```python
from build123d import *

# Parameters (mm, degrees)
SKETCH1_R            = 15
BOSS_EXTRUDE1_DEPTH  = 40
SKETCH2_R            = 35
BOSS_EXTRUDE2_DEPTH  = 5
SKETCH3_R            = 5
CUT_EXTRUDE1_DEPTH   = 64.639610307
CUT_EXTRUDE2_DEPTH   = 10
SKETCH5_W            = 7.5
SKETCH5_H            = 12
CUT_EXTRUDE3_DEPTH   = 64.639610307
M5_CLEARANCE_HOLE1_D = 5.5
CUT_EXTRUDE4_DEPTH   = 64.639610307


with BuildPart() as part:
    # Sketch1 → Boss-Extrude1 (new body)
    with BuildSketch(Plane.XY):
        Circle(SKETCH1_R)
    extrude(amount=BOSS_EXTRUDE1_DEPTH)

    # Sketch2 → Boss-Extrude2 (add)
    with BuildSketch(Plane(origin=(0, 0, 0), x_dir=(-1, 0, 0), z_dir=(0, 0, -1))):
        Circle(SKETCH2_R)
    extrude(amount=-BOSS_EXTRUDE2_DEPTH)

    # Sketch3 → Cut-Extrude1 (cut, through all)
    with BuildSketch(Plane(origin=(0, 0, 0), x_dir=(-1, 0, 0), z_dir=(0, 0, -1))):
        Circle(SKETCH3_R)
    extrude(amount=-CUT_EXTRUDE1_DEPTH, mode=Mode.SUBTRACT)

    # Sketch4 → Cut-Extrude2 (cut)
    with BuildSketch(Plane(origin=(0, 0, 0), x_dir=(-1, 0, 0), z_dir=(0, 0, -1))):
        Polygon((8, 0), (4, 6.92820323), (-4, 6.92820323), (-8, 0), (-4, -6.92820323), (4, -6.92820323), align=None)
    extrude(amount=-CUT_EXTRUDE2_DEPTH, mode=Mode.SUBTRACT)

    # Sketch5 → Cut-Extrude3 (cut, symmetric)
    with BuildSketch(Plane(origin=(0, 0, 0), x_dir=(1, 0, 0), z_dir=(0, 1, 0))):
        with Locations((11.25, -34)):
            Rectangle(SKETCH5_W, SKETCH5_H)
    cut_extrude3 = extrude(amount=CUT_EXTRUDE3_DEPTH, both=True, mode=Mode.SUBTRACT)

    # Mirror1: Cut-Extrude3 across plane
    add(cut_extrude3.mirror(Plane(origin=(0, 0, 0), x_dir=(0, 0, 1), z_dir=(1, 0, 0))), mode=Mode.SUBTRACT)

    # M5 Clearance Hole1 (through all)
    with Locations(Plane(origin=(0, 0, 0), x_dir=(-1, 0, 0), z_dir=(0, 0, -1))):
        with Locations((0, 27.5), (-27.5, 0), (27.5, 0), (0, -27.5)):
            Hole(M5_CLEARANCE_HOLE1_D / 2)

    # Sketch8 → Cut-Extrude4 (cut, through all)
    with BuildSketch(Plane(origin=(0, 0, 0), x_dir=(-1, 0, 0), z_dir=(0, 0, -1))):
        with BuildLine():
            Line((-34.957538249, -1.723519533), (1.723519533, 34.957538249))
            ThreePointArc((1.723519533, 34.957538249), (-24.748737342, 24.748737342), (-34.957538249, -1.723519533))
        make_face()
    extrude(amount=-CUT_EXTRUDE4_DEPTH, mode=Mode.SUBTRACT)


solid = part.part
```
Read the model definition and answer for the solid it produces. Units are mm, in the model's axes. A direction names the side the tool comes from. Coordinates: 2 decimals unless noted, no trailing zeros. Loops run counter-clockwise (first coordinate to the right, second up) from the corner with the lowest first, then second, coordinate; pieces in that order, holes last. Notation, with made-up numbers: (-28.75, 15.25) - (-24.75, 15.25) arc R16 cw to (-24.75, 24.25) - close; hole circle Ø11 at (80.5, 3). An arc over 180 degrees is marked (long way). Answer in a Markdown table with one row per item.
1. Given pin 1 (4 mm diameter, centred on y = 17, z = 4, fed in from +X); pin 2 (3 mm diameter, centred on y = 2, z = 24.5, fed in from +X); pin 3 (6 mm diameter, centred on x = 13, y = 5, fed in from +Z), each flat-ended and moving along its own axis, determine where each tip first touches the part or whether it passes through.
Conclusion:
| item | result |
|---|---|
| pin 1 | stops at x = 18.23 |
| pin 2 | stops at x = 14.99 |
| pin 3 | stops at z = 28 |
2. Straight lines are drawn through the part: line 1 (Y direction, x = 0, z = 4); line 2 (Z direction, x = -18, y = 18); line 3 (X direction, y = -4, z = 14). For each, find the intervals that lie inside material, in ascending order.
Conclusion:
| item | result |
|---|---|
| line 1 | y = -35 to -30.25, -24.75 to -6.93, 6.93 to 24.75, 30.25 to 33.23 |
| line 2 | z = 0 to 5 |
| line 3 | x = -14.46 to -3, 3 to 14.46 |
3. Find section B-B, the plane x = -27.5. Write down the section's boundary in (y, z), then the cut area to 3 significant figures.
Conclusion:
| item | result |
|---|---|
| outline | (-21.65, 0) - (-2.75, 0) - (-2.75, 5) - (-21.65, 5) - close; (2.75, 0) - (21.65, 0) - (21.65, 5) - (2.75, 5) - close |
| area | 189 mm² |
4. Determine the mould class of faces 1 (the face through (-7.5, 0, 34)), 2 (the face through (-0.358, 30.227, 2.535)), 3 (the face through (10, 0, 28)) for opening direction X: +X half, -X half, draft (parallel to the pull), parting line (faces both ways), or undercut.
Conclusion:
| item | result |
|---|---|
| face 1 | -X half |
| face 2 | undercut |
| face 3 | draft |
5. Find section D-D, the plane z = 34. Write down the section's boundary in (x, y).
Conclusion:
| item | result |
|---|---|
| outline | (-7.5, -12.99) arc R15 ccw to (7.5, -12.99) - (7.5, 12.99) arc R15 ccw to (-7.5, 12.99) - close; hole circle Ø10 at (0, 0) |
6. Find section A-A, the plane z = 3.5. Write down the section's boundary in (x, y).
Conclusion:
| item | result |
|---|---|
| outline | (-1.72, 34.96) arc R35 ccw (long way) to (34.96, -1.72) - close; hole circle Ø5.5 at (-27.5, 0); hole (-8, 0) - (-4, -6.93) - (4, -6.93) - (8, 0) - (4, 6.93) - (-4, 6.93) - close; hole circle Ø5.5 at (0, -27.5); hole circle Ø5.5 at (0, 27.5); hole circle Ø5.5 at (27.5, 0) |
7. Find section C-C, the plane y = 27.5. Write down the section's boundary in (x, z).
Conclusion:
| item | result |
|---|---|
| outline | (-21.65, 0) - (-2.75, 0) - (-2.75, 5) - (-21.65, 5) - close; (2.75, 0) - (5.73, 0) - (5.73, 5) - (2.75, 5) - close |
8. Which of the six approach directions +Z, -Z, +X, -X, +Y, -Y give full straight-line access (tool end or side, diameter ignored) to faces 4 (the face through (-5, -3, 40)), 5 (the face through (-10, 0, 28)), 6 (the face through (-15, -7, 5)), 7 (the face through (6.028, -3.416, 4.93))?
Conclusion:
| item | result |
|---|---|
| face 4 | +Z, +X, -X, +Y, -Y |
| face 5 | +Z, -X, +Y, -Y |
| face 6 | +Z |
| face 7 | -Z |
